Autodesk Inventor part; units mm, degrees
ref_plane "YZ Plane" through (0, 0, 0) normal (1, 0, 0) x (0, 1, 0)
ref_plane "XZ Plane" through (0, 0, 0) normal (0, 1, 0) x (-1, 0, 0)
ref_plane "XY Plane" through (0, 0, 0) normal (0, 0, 1) x (1, 0, 0)
sketch "Sketch1" plane through (0, 0, 0) normal (0, 1, 0) x (-1, 0, 0)
  line L0 (-51.9733, 36.6301) -> (-51.9733, 68.3801)
  line L1 (-65.3083, 74.7301) -> (-65.3083, 36.6301)
  line L2 (-65.3083, 36.6301) -> (-62.1333, 36.6301)
  line L3 (-62.1333, 36.6301) -> (-62.1333, 62.0301)
  line L4 (-62.1333, 62.0301) -> (-57.0533, 62.0301)
  line L5 (-57.0533, 62.0301) -> (-57.0533, 36.6301)
  line L6 (-57.0533, 36.6301) -> (-51.9733, 36.6301)
  line L7 (-51.9733, 68.3801) -> (-20.8583, 68.3801)
  line L8 (-20.8583, 68.3801) -> (-20.8583, 74.7301)
  line L9 (-20.8583, 74.7301) -> (-65.3083, 74.7301)
  dimension "d2" = 5.08
  dimension "d4" = 25.4
  dimension "d18" = 6.35
  dimension "d19" = 38.1
  dimension "d20" = 3.175
  dimension "d79" = 5.08
  dimension "d80" = 44.45
extrude "Extrusion1" add sketch "Sketch1" along normal blind 177.8
ref_plane "Work Plane2" through (65.3083, -38.1, 36.6301) normal (1, 0, 0) x (0, 0, -1)
sketch "Sketch13" plane through (20.8583, 0, 74.7301) normal (0, 0, 1) x (1, 0, 0)
  line L0 (38.1, 0) -> (44.45, 0)
  line L1 (44.45, 0) -> (44.45, 177.8)
  line L2 (44.45, 177.8) -> (38.1, 177.8)
  line L3 (38.1, 177.8) -> (38.1, 0)
  line L4 (44.45, 0) -> (44.45, 177.8)
  line L5 (0, 177.8) -> (44.45, 177.8)
  line L6 (0, 0) -> (44.45, 0)
  point P0 (-20.8583, 0)
  point P1 (36.195, 177.8)
  point P2 (41.275, 177.8)
  point P3 (36.195, 0)
  point P4 (41.275, 0)
  point P5 (31.115, 0)
  dimension "d81" = 6.35
extrude "Extrusion2" add sketch "Sketch13" along normal blind 50.8
sketch "Sketch21" plane through (58.9583, 0, 74.7301) normal (-1, 0, 0) x (0, 0, 1)
  line L0 (50.8, 177.8) -> (50.8, 0)
  line L1 (50.8, 0) -> (44.45, 0)
  line L2 (44.45, 0) -> (44.45, 177.8)
  line L3 (44.45, 177.8) -> (50.8, 177.8)
  line L4 (50.8, 177.8) -> (50.8, 0)
  line L5 (0, 177.8) -> (50.8, 177.8)
  point P0 (-74.7301, 0)
  dimension "d91" = 6.35
extrude "Extrusion10" add sketch "Sketch21" along normal blind 38.1
sketch "Sketch22" plane through (51.9733, 0, 68.3801) normal (0, 0, -1) x (-1, 0, 0)
  line L0 (31.115, 0) -> (31.115, 177.8)
  line L1 (0, 44.45) -> (31.115, 44.45)
  line L2 (31.115, 44.45) -> (31.115, 133.35)
  line L3 (31.115, 133.35) -> (0, 133.35)
  line L4 (0, 133.35) -> (0, 44.45)
  line L5 (0, 0) -> (31.115, 0)
  line L6 (0, 177.8) -> (31.115, 177.8)
  line L7 (0, 0) -> (0, 177.8)
  point P0 (51.9733, 0)
  dimension "d94" = 44.45
  dimension "d95" = 44.45
extrude "Extrusion11" cut sketch "Sketch22" against normal blind 76.2 contours L1 L4 L3 L0
sketch "Sketch23" plane through (20.8583, 0, 74.7301) normal (0, 0, 1) x (1, 0, 0)
  line L0 (0, 177.8) -> (38.1, 177.8)
  line L1 (38.1, 177.8) -> (31.115, 177.8)
  line L2 (31.115, 177.8) -> (31.115, 0)
  line L3 (31.115, 0) -> (38.1, 0)
  line L4 (38.1, 0) -> (38.1, 177.8)
  line L5 (31.115, 133.35) -> (31.115, 44.45)
  line L6 (38.1, 0) -> (38.1, 177.8)
  line L7 (0, 0) -> (38.1, 0)
  point P0 (-20.8583, 0)
revolve "Revolution8" add sketch "Sketch23" angle 90 about axis through (58.9583, 0, 74.7301) along (0, 1, 0)
sketch "Sketch24" plane through (58.9583, 0, 119.1801) normal (0, 0, -1) x (-1, 0, 0)
  line L0 (0, 0) -> (0, 177.8)
  line L1 (0, 177.8) -> (38.1, 177.8)
  line L2 (0, 0) -> (6.985, 0)
  line L3 (6.985, 0) -> (6.985, 177.8)
  line L4 (6.985, 177.8) -> (0, 177.8)
  line L5 (0, 177.8) -> (0, 0)
  line L6 (6.985, 44.45) -> (6.985, 133.35)
  point P0 (58.9583, 0)
revolve "Revolution9" add sketch "Sketch24" angle 90 about axis through (58.9583, 177.8, 119.1801) along (0, -1, 0)
sketch "Sketch25" plane through (65.3083, 0, 36.6301) normal (1, 0, 0) x (0, 0, -1)
  line L0 (-38.1, 44.45) -> (-82.55, 44.45)
  line L1 (-82.55, 44.45) -> (-82.55, 133.35)
  line L2 (-82.55, 133.35) -> (-38.1, 133.35)
  line L3 (-38.1, 133.35) -> (-38.1, 44.45)
  line L4 (-88.9, 0) -> (-88.9, 177.8)
  line L5 (-38.1, 133.35) -> (-38.1, 44.45)
  line L6 (0, 0) -> (-88.9, 0)
  line L7 (0, 177.8) -> (-88.9, 177.8)
  line L8 (-82.55, 44.45) -> (-82.55, 0)
  point P0 (36.6301, 0)
  dimension "d100" = 44.45
  dimension "d101" = 44.45
extrude "Extrusion12" cut sketch "Sketch25" against normal blind 76.2
sketch "Sketch26" plane through (65.3083, 0, 36.6301) normal (1, 0, 0) x (0, 0, -1)
  line L0 (0, 177.8) -> (0, 0)
  line L1 (0, 88.9) -> (-55.1771, 88.9)
  line L2 (0, 0) -> (0, 177.8)
  line L3 (0, 177.8) -> (-88.9, 177.8)
  line L4 (0, 0) -> (-88.9, 0)
  line L5 (-25.4, 0) -> (-25.4, 177.8)
  point P0 (36.6301, 0)
  point P1 (-12.7, 158.75)
  point P2 (-12.7, 107.95)
  point P3 (-12.7, 69.85)
  point P4 (-12.7, 19.05)
  dimension "d104" = 19.05
  dimension "d105" = 19.05
  dimension "d106" = 69.85
  dimension "d107" = 69.85
  dimension "d108" = 12.7
  dimension "d109" = 12.7
  dimension "d110" = 12.7
  dimension "d111" = 12.7
hole "Hole4" at (65.3083, 19.05, 49.3301) at (65.3083, 69.85, 49.3301) at (65.3083, 107.95, 49.3301) at (65.3083, 158.75, 49.3301) direction (-1, 0, 0) diameter 6.35 end through all
sketch "Sketch27" plane through (65.3083, 0, 36.6301) normal (1, 0, 0) x (0, 0, -1)
  line L0 (0, 0) -> (0, 177.8)
  line L1 (0, 88.9) -> (-38.1, 88.9)
  line L2 (-38.1, 133.35) -> (-38.1, 44.45)
  line L3 (-17.4625, 88.9) -> (-17.4625, 82.55)
  line L4 (-17.4625, 82.55) -> (-4.7625, 82.55)
  line L5 (-4.7625, 82.55) -> (-4.7625, 88.9)
  line L6 (-17.4625, 38.1) -> (-4.7625, 38.1)
  line L7 (-4.7625, 38.1) -> (-4.7625, 50.8)
  line L8 (-4.7625, 50.8) -> (-17.4625, 50.8)
  line L9 (-17.4625, 50.8) -> (-17.4625, 38.1)
  line L10 (-17.4625, 88.9) -> (-17.4625, 95.25)
  line L11 (-17.4625, 95.25) -> (-4.7625, 95.25)
  line L12 (-4.7625, 95.25) -> (-4.7625, 88.9)
  line L13 (-17.4625, 139.7) -> (-4.7625, 139.7)
  line L14 (-4.7625, 139.7) -> (-4.7625, 127)
  line L15 (-4.7625, 127) -> (-17.4625, 127)
  line L16 (-17.4625, 127) -> (-17.4625, 139.7)
  point P0 (36.6301, 0)
  dimension "d119" = 12.7
  dimension "d120" = 6.35
  dimension "d121" = 31.75
  dimension "d122" = 12.7
  dimension "d123" = 12.7
extrude "Extrusion13" cut sketch "Sketch27" against normal blind 25.4
sketch "Sketch28" plane through (51.9733, 0, 68.3801) normal (0, 0, -1) x (-1, 0, 0)
  circle A0 centre (12.065, 22.225) radius 6.35
  line L0 (31.115, 0) -> (31.115, 44.45)
  line L1 (31.115, 44.45) -> (0, 44.45)
  circle A1 centre (12.065, 155.575) radius 6.35
  line L2 (31.115, 133.35) -> (31.115, 177.8)
  line L3 (0, 133.35) -> (31.115, 133.35)
  point P0 (51.9733, 0)
  dimension "d126" = 12.7
  dimension "d127" = 19.05
  dimension "d128" = 22.225
  dimension "d129" = 12.7
  dimension "d130" = 19.05
  dimension "d131" = 22.225
extrude "Extrusion14" cut sketch "Sketch28" against normal through all
properties part number "Suspension mount 2.0" material "Acetal Resin, Black"
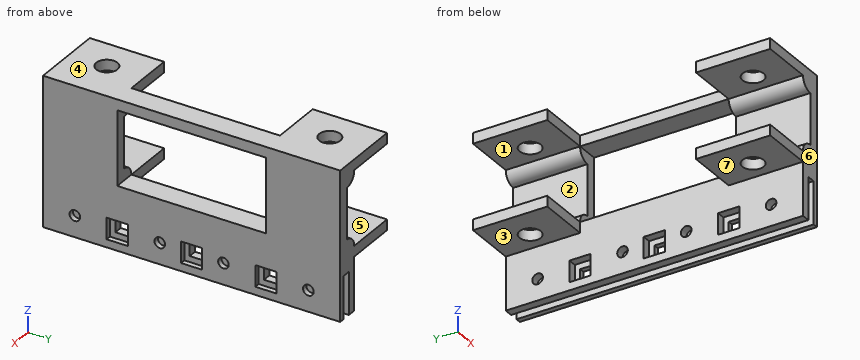
The model under review builds one solid part; all positions refer to its coordinate system, in mm. Face numbers are marked on the shaded views. A direction names the side the tool comes from. Round coordinates to 2 decimals unless told otherwise and drop trailing zeros. Order: outer loops, then holes, each group sorted by start corner. A loop starts at its lowest first (then second) coordinate and runs counter-clockwise, first axis right, second up. Notation, with made-up numbers: (-6, 66.5) -> (16, 66.5) arc R34 cw to (16, 104.5) -> close; hole circle Ø3 at (50.25, 53). An arc over 180 degrees is marked (long way). Write item = value, one per line. Start each with the question number.
Item 1: For the marked faces 5, 6 and 7, list the 3-axis set-ups (+Z, -Z, +X, -X, +Y, -Y) from which the entire face can be reached by the end or side of a thin tool; tool diameter is ignored.
Item 2: For line 1 along Z through (x, y) = (63.8, 107.95); line 2 along X through (y, z) = (158.5, 44.5); line 3 along Z through (x, y) = (39, 10), list the stretches that pass through material, from the lowest coordinate up.
Item 3: Consider section B-B on z = 103.5. Write out the cut boundary in (x, y), plus the area to 3 significant figures.
Item 4: Consider section D-D on y = 131. Write out the cut boundary in (x, z), plus the area to 3 significant figures.
Item 5: Clearance check with flat-ended pins moving along their axes: pin 1 Ø5.5 at (y, z) = (69.85, 49.33) entering from +X; pin 2 Ø15 at (y, z) = (25.5, 91) entering from -X. State where each tip first meets the part, or that it passes through.
Item 6: Consider section C-C on x = 24. Write out the cut boundary in (y, z).
Item 7: Consider section A-A on y = 107.95. Write out the cut boundary in (x, z), plus the area to 3 significant figures.
Item 8: Mouldability with a two-part tool opening along Z and no side actions: class the marked faces 1, 2, 3 and 4 as released by +Z, released by -Z, zero draft, split by the parting line, or undercut.
Conclusion:
q1.face_5 = -X, +Y, -Y
q1.face_6 = +Z, -Z, +X, -X, -Y
q1.face_7 = -Z, -X, +Y, -Y
q2.line_1 = 36.63 to 46.16, 52.51 to 74.73, 119.18 to 125.53
q2.line_2 = 51.97 to 57.05, 62.13 to 65.31
q2.line_3 = 68.38 to 74.73, 119.18 to 125.53
q3.outline = (58.96, 0) -> (65.31, 0) -> (65.31, 44.45) -> (58.96, 44.45) -> close; (58.96, 133.35) -> (65.31, 133.35) -> (65.31, 177.8) -> (58.96, 177.8) -> close
q3.area = 565 mm2
q4.outline = (51.97, 36.63) -> (57.05, 36.63) -> (57.05, 41.39) -> (51.97, 41.39) -> close; (51.97, 54.09) -> (57.05, 54.09) -> (57.05, 62.03) -> (62.13, 62.03) -> (62.13, 54.09) -> (65.31, 54.09) -> (65.31, 74.73) -> (51.97, 74.73) -> close; (51.97, 119.18) -> (65.31, 119.18) -> (65.31, 125.53) -> (51.97, 125.53) -> close; (62.13, 36.63) -> (65.31, 36.63) -> (65.31, 41.39) -> (62.13, 41.39) -> close
q4.area = 359 mm2
q5.pin_1 = through
q5.pin_2 = 58.96
q6.outline = (0, 68.38) -> (44.45, 68.38) -> (44.45, 74.73) -> (0, 74.73) -> close; (0, 119.18) -> (44.45, 119.18) -> (44.45, 125.53) -> (0, 125.53) -> close; (133.35, 68.38) -> (177.8, 68.38) -> (177.8, 74.73) -> (133.35, 74.73) -> close; (133.35, 119.18) -> (177.8, 119.18) -> (177.8, 125.53) -> (133.35, 125.53) -> close
q7.outline = (51.97, 36.63) -> (57.05, 36.63) -> (57.05, 46.16) -> (51.97, 46.16) -> close; (51.97, 52.51) -> (57.05, 52.51) -> (57.05, 62.03) -> (62.13, 62.03) -> (62.13, 52.51) -> (65.31, 52.51) -> (65.31, 74.73) -> (51.97, 74.73) -> close; (51.97, 119.18) -> (65.31, 119.18) -> (65.31, 125.53) -> (51.97, 125.53) -> close; (62.13, 36.63) -> (65.31, 36.63) -> (65.31, 46.16) -> (62.13, 46.16) -> close
q7.area = 411 mm2
q8.face_1 = undercut
q8.face_2 = undercut
q8.face_3 = released by -Z
q8.face_4 = released by +Z
